Here's how the part is built. I have some questions about the finished solid (model axes, mm). A direction names the side the tool comes from. Coordinates: 2 decimals unless noted, no trailing zeros. Write each loop counter-clockwise with the first axis right and the second up, starting at its lowest first coordinate (ties: lowest second). Pieces come first, ordered by that corner, then holes. Notation, with made-up numbers: (-25, 67.25) -> (-11, 67.25) arc R20 ccw to (-11, 80.25) -> close; hole circle Ø10 at (-18.75, -16.75). An arc over 180 degrees is marked (long way). Use a Markdown table: item, result. Add a question column.
Item 1: If we mould it in two halves opening along Z, with no side actions, what happens to faces 3 (the flat face through (0, -1, -24)), 4 (the cylindrical face through (-11.878, 4.54, -18.777)), 5 (the flat face through (0, -1, 24)), 6 (the flat face through (0, -3, 6))? For each: pulls with the +Z half, pulls with the -Z half, needs draft (parallel to the pull), parting line crosses it, or undercut.
Item 2: Will these pins go through, and if not, where does the flat tip stop? pin 1 Ø12 at (y, z) = (30, -17) entering from +X; pin 2 Ø5 at (y, z) = (11.5, -2.5) entering from -X; pin 3 Ø12 at (x, z) = (26, 15) entering from +Y.
Item 3: Imagine slicing it at B-B, the plane z = 0. Write out the boundary of the cut face in (x, y).
Item 4: Imagine slicing it at A-A, the plane x = 0. Write out the boundary of the cut face in (y, z), and give its area (3 significant figures).
Item 5: Imagine slicing it at C-C, the plane y = 26.5. Write out the boundary of the cut face in (x, z), and give its area (3 significant figures).
Item 6: If I drill on line 1 along Z through (x, y) = (0, -1); line 2 along X through (y, z) = (-2.1, 0); line 3 along Y through (x, z) = (4.5, -5), over which ranges is the centre line in solid material (lowest first)? Write a range as from..to.
Item 7: On a 3-axis mill with a long thin cutter (end or side, diameter ignored), from which of +Z, -Z, +X, -X, +Y, -Y can I reach the whole of each face in a straight line? I mean faces 1 (the flat face through (0, 0, 6)), 2 (the cylindrical face through (29.555, 35.159, -18.777)). Say none if no direction works.
```python
from build123d import *

# Parameters (mm, degrees)
BOSS_EXTRU_1_DEPTH      = 48
BOSS_EXTRU_1_DEPTH_BACK = 48
ESQUISSE2_R             = 2.2
ENL_V_MAT_EXTRU_1_DEPTH = 10
CONG_1_R                = 25
ECHELLE1_SCALE          = 0.5
ESQUISSE3_R             = 5
ENL_V_MAT_EXTRU_2_DEPTH = 10


with BuildPart() as part:
    # Esquisse1 → Boss.-Extru.1 (new body, two sides)
    with BuildSketch(Plane.XY) as boss_extru_1_sk:
        Polygon((15, 0), (-15, 0), (-62.5, 82.27241336), (-67.696152423, 79.27241336), (-18.464101615, -6), (18.464101615, -6), (67.696152423, 79.27241336), (62.5, 82.27241336), align=None)
    extrude(amount=BOSS_EXTRU_1_DEPTH)
    extrude(boss_extru_1_sk.sketch, amount=-BOSS_EXTRU_1_DEPTH_BACK)

    # Esquisse2 → Enl_v. mat.-Extru.1 (cut)
    with BuildSketch(Plane(origin=(-16.446152423, -9.495190528, 0), x_dir=(0, 0, 1), z_dir=(-0.866025404, -0.5, 0))):
        with Locations((-35.355339059, 19.644660941)):
            Circle(ESQUISSE2_R)
        with Locations((35.355339059, 90.355339059)):
            Circle(ESQUISSE2_R)
        with Locations((35.355339059, 19.644660941)):
            Circle(ESQUISSE2_R)
        with Locations((-35.355339059, 90.355339059)):
            Circle(ESQUISSE2_R)
    enl_v_mat_extru_1 = extrude(amount=-ENL_V_MAT_EXTRU_1_DEPTH, mode=Mode.SUBTRACT)

    # Cong_1
    cong_1_edges = [part.edges().sort_by_distance(p)[0] for p in [
        (-65.098076211, 80.77241336, 48),
        (65.098076211, 80.77241336, -48),
        (65.098076211, 80.77241336, 48),
        (-65.098076211, 80.77241336, -48),
    ]]
    fillet(cong_1_edges, radius=CONG_1_R)

    # Sym_trie1: Enl_v. mat.-Extru.1 across plane
    add(enl_v_mat_extru_1.mirror(Plane(origin=(0, 0, 0), x_dir=(0, 0, 1), z_dir=(1, 0, 0))), mode=Mode.SUBTRACT)


with BuildPart() as part_1:
    # Echelle1: scaled about (0, 0, 0)
    add(part.part.scale(ECHELLE1_SCALE))

    # Esquisse3 → Enl_v. mat.-Extru.2 (cut)
    with BuildSketch(Plane(origin=(0, 0, 0), x_dir=(1, 0, 0), z_dir=(0, 1, 0))):
        Circle(ESQUISSE3_R)
    extrude(amount=-ENL_V_MAT_EXTRU_2_DEPTH, mode=Mode.SUBTRACT)


solid = part_1.part
```
Ans:
| question | item | result |
|---|---|---|
| 1 | face 3 | pulls with the -Z half |
| 1 | face 4 | undercut |
| 1 | face 5 | pulls with the +Z half |
| 1 | face 6 | needs draft |
| 2 | pin 1 | stops at x = 31.75 |
| 2 | pin 2 | stops at x = -19.05 |
| 2 | pin 3 | stops at y = 41.12 |
| 3 | outline | (-33.85, 39.64) -> (-9.23, -3) -> (-5, -3) -> (-5, 0) -> (-7.5, 0) -> (-31.25, 41.14) -> close; (5, -3) -> (9.23, -3) -> (33.85, 39.64) -> (31.25, 41.14) -> (7.5, 0) -> (5, 0) -> close |
| 4 | outline | (-3, -24) -> (0, -24) -> (0, -5) -> (-3, -5) -> close; (-3, 5) -> (0, 5) -> (0, 24) -> (-3, 24) -> close |
| 4 | area | 114 mm^2 |
| 5 | outline | (-26.26, -24) -> (-22.8, -24) -> (-22.8, 24) -> (-26.26, 24) -> close; (22.8, -24) -> (26.26, -24) -> (26.26, 24) -> (22.8, 24) -> close |
| 5 | area | 333 mm^2 |
| 6 | line 1 | z = -24..-5, 5..24 |
| 6 | line 2 | x = -9.75..-5, 5..9.75 |
| 6 | line 3 | y = -3..0 |
| 7 | face 1 | +Z, -Z, +Y |
| 7 | face 2 | none |
